Work out the finished part from the listing and answer in its coordinate system (mm). Coordinates: 2 decimals unless noted, no trailing zeros. Loops run counter-clockwise (first coordinate to the right, second up) from the corner with the lowest first, then second, coordinate; pieces in that order, holes last. Notation, with made-up numbers: (-10, -21.5) - (19, -21.5) arc R16 cw to (19, -1.5) - close; hole circle Ø1 at (88, 69.25). An arc over 180 degrees is marked (long way). Write each question's results on one line, items separated by ' | '. Start each with the question number.
Item 1: Consider probe 1 along X at (y, z) = (-14, 20.5); probe 2 along Z at (x, y) = (31, -3.5); probe 3 along X at (y, z) = (-31, 23). Determine where each line is inside the solid, lowest interval first. Write a range as [from, to].
Item 2: Section B-B, the plane x = 486 is taken. Write down the section's boundary in (y, z).
Item 3: Section A-A, the plane y = -9 is taken. Write down the section's boundary in (x, z), plus the area to 3 significant figures.
Item 4: Each of these flat-tipped pins is pushed along its axis until it touches: pin 1 Ø2 at (x, y) = (1100, -17.5) entering from -Z; pin 2 Ø10 at (x, y) = (255.5, -4.5) entering from -Z. Where does it stop, or does it pass through?
Item 5: Section C-C, the plane x = 1087.5 is taken. Write down the section's boundary in (y, z), plus the area to 3 significant figures.
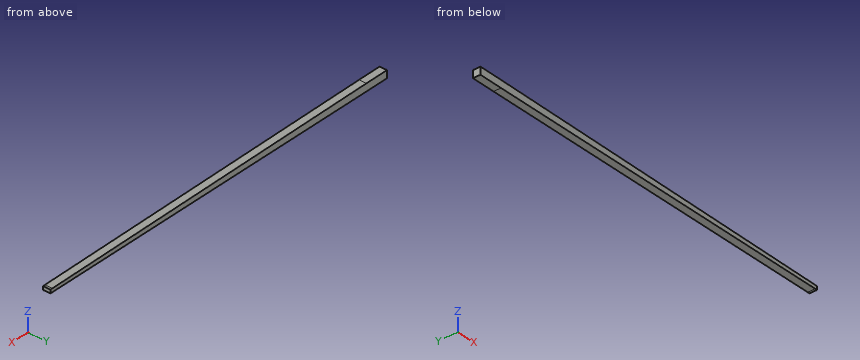
from build123d import *

# Parameters (mm, degrees)
F1_DEPTH = 43.18
F2_W     = 43.18
F2_H     = 43.18
F3_DEPTH = 139.7
F4_W     = 43.18
F4_H     = 20.32
F5_DEPTH = 12.7


with BuildPart() as f1:
    # F0 (on Front) → F1 (new body)
    with BuildSketch(Plane.XZ):
        Polygon((0, 43.18), (0, 0), (2133.6, 10.16), (2133.503239, 30.47977), align=None)
    extrude(amount=F1_DEPTH)

    # F2 (on face) → F3 (join)
    with BuildSketch(Plane(origin=(0, 0, 0), x_dir=(0, -1, 0), z_dir=(-1, 0, 0))):
        with Locations((21.59, 21.59)):
            Rectangle(F2_W, F2_H)
    extrude(amount=F3_DEPTH)

    # F4 (on face) → F5 (join)
    with BuildSketch(Plane(origin=(2133.6, 0, 10.16), x_dir=(0, 1, 0), z_dir=(0.999989, 0, 0.004762))):
        with Locations((-21.59, 10.16)):
            Rectangle(F4_W, F4_H)
    extrude(amount=F5_DEPTH)


solid = f1.part
Answer key:
1) probe 1: x = [-139.7, 2146.25] | probe 2: z = [0.15, 43] | probe 3: x = [-139.7, 2146.24]
2) outline: (-43.18, 2.31) - (0, 2.31) - (0, 40.29) - (-43.18, 40.29) - close
3) outline: (-139.7, 0) - (0, 0) - (2133.6, 10.16) - (2146.3, 10.22) - (2146.2, 30.54) - (2133.5, 30.48) - (0, 43.18) - (-139.7, 43.18) - close | area: 74,000 mm^2
4) pin 1: stops at z = 5.23 | pin 2: stops at z = 1.19
5) outline: (-43.18, 5.18) - (0, 5.18) - (0, 36.71) - (-43.18, 36.71) - close | area: 1,360 mm^2
